Study the drawing (mm; zero at the part's minimum x, y, z) and answer. Give positions to 0.01 mm unless a question says otherwise; leave off trailing zeros. Order: outer loops, then holes, each group sorted by start corner. A loop starts at its lowest first (then second) coordinate and runs counter-clockwise, first axis right, second up. Notation, with made-up numbers: (46.25, 82.25) - (54.25, 82.25) arc R16 cw to (54.25, 99.25) - close; hole circle Ø1 at (11, 17.25). An arc over 180 degrees is marked (long way). Return JSON: item names as keys, results as strings.
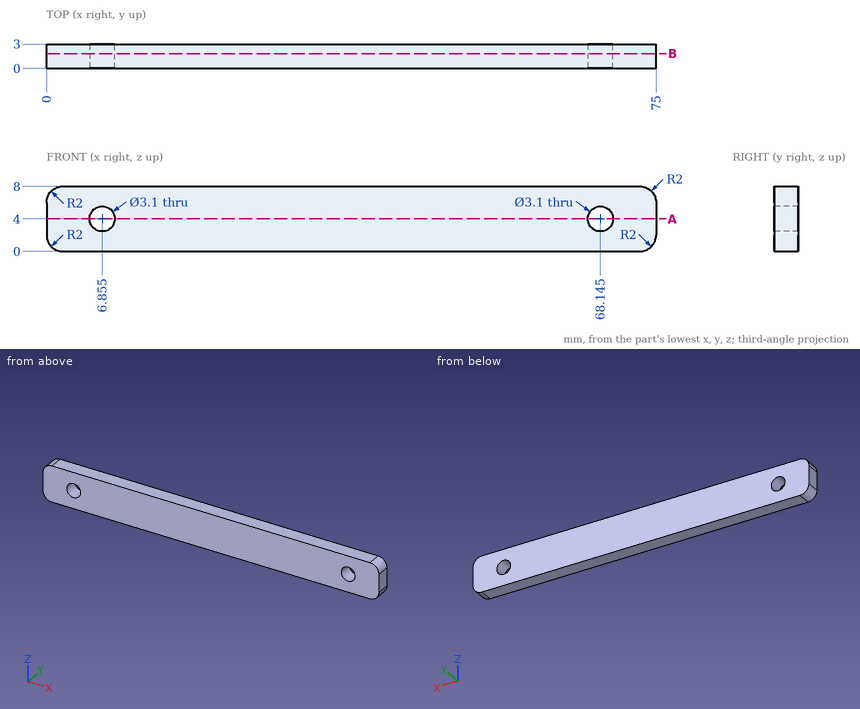
Q1. Consider L1, parallel to X at y = 1.75, z = 4 (3 decimals); L2, parallel to Z at x = 68, y = 2.5; L3, parallel to X at y = 0.35, z = 3.25. Determine where each line is inside the solid, lowest interval first.
Values:
{"L1": "x = 0 to 5.305, 8.405 to 66.595, 69.695 to 75", "L2": "z = 0 to 2.46, 5.54 to 8", "L3": "x = 0 to 5.5, 8.21 to 66.79, 69.5 to 75"}
Q2. A cutting plane is placed at A-A (z = 4). Write down the section's boundary in (x, y) (3 decimals), and give its area (3 significant figures).
Values:
{"outline": "(0, 0) - (5.305, 0) - (5.305, 3) - (0, 3) - close; (8.405, 0) - (66.595, 0) - (66.595, 3) - (8.405, 3) - close; (69.695, 0) - (75, 0) - (75, 3) - (69.695, 3) - close", "area": "206 mm²"}
Q3. Given pin 1 (2.5 mm diameter, centred on x = 6.855, z = 4, fed in from -Y), flat-ended and moving along its own axis, determine where the tip first touches the part or whether it passes through.
Values:
{"pin 1": "passes through"}
Q4. A cutting plane is placed at B-B (y = 1.8). Write down the section's boundary in (x, z) (3 decimals), and give its area (3 significant figures).
Values:
{"outline": "(0, 2) arc R2 ccw to (2, 0) - (73, 0) arc R2 ccw to (75, 2) - (75, 6) arc R2 ccw to (73, 8) - (2, 8) arc R2 ccw to (0, 6) - close; hole circle Ø3.1 at (6.855, 4); hole circle Ø3.1 at (68.145, 4)", "area": "581 mm²"}
